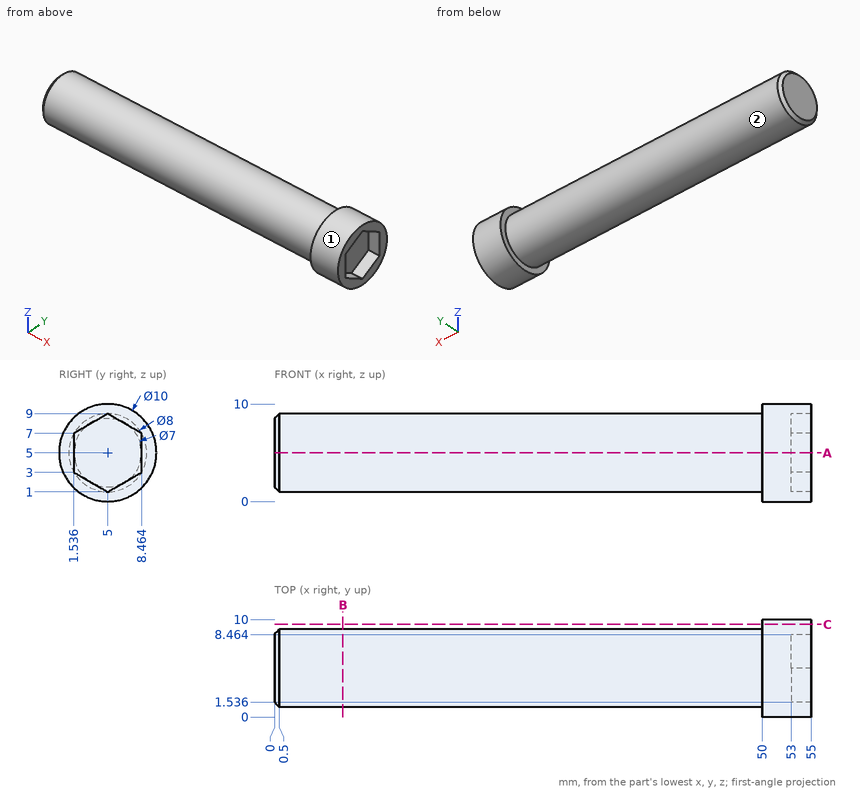
Geometry check sheet. Reference: drawing and pictorial views, mm from the part's lowest x, y, z. A direction names the side the tool comes from. Coordinates: 2 decimals unless noted, no trailing zeros. Order: outer loops, then holes, each group sorted by start corner. A loop starts at its lowest first (then second) coordinate and runs counter-clockwise, first axis right, second up. Notation, with made-up numbers: (-25, 85.25) -> (27, 85.25) arc R21 cw to (27, 110.25) -> close; hole circle Ø9 at (36, 55.25). An arc over 180 degrees is marked (long way). Use CSV: the item, a comma, the result in double quotes. Start each with the question number.
Q1. Section check B-B, the plane x = 7. Record the cut outline in (y, z).
Q2. Section check A-A, the plane z = 5. Record the cut outline in (x, y).
Q3. Tool access check on the marked faces 1 and 2. Record the directions out of +Z, -Z, +X, -X, +Y, -Y that give a thin tool (end or side, any length) a straight path to the whole face; none if there is none.
Q4. Section check C-C, the plane y = 9.5. Record the cut outline in (x, z), and give its area (3 significant figures).
Q5. Thickness scan on line 1 along X through (y, z) = (3.5, 2.25); line 2 along X through (y, z) = (9, 6.25); line 3 along Z through (x, y) = (40, 5.25). Record the ranges inside material, lowest first.
Q6. Depth check by flat-ended pin: P1, Ø2, axis at x = 16.5, y = 2.5, coming from the -Z side; P2, Ø5.5, axis at y = 4.5, z = 4, coming from the +X side; P3, Ø6, axis at x = 45, z = 5, coming from the +Y side; P4, Ø0.6, axis at x = 54.5, z = 5.5, coming from the -Y side. Enter the tip coordinate at first touch or a pass-through.
Returned:
1,outline,"circle Ø8 at (5, 5)"
2,outline,"(0, 1.5) -> (0.5, 1) -> (50, 1) -> (50, 0) -> (55, 0) -> (55, 1.54) -> (53, 1.54) -> (53, 8.46) -> (55, 8.46) -> (55, 10) -> (50, 10) -> (50, 9) -> (0.5, 9) -> (0, 8.5) -> close"
3,face 1,"+X, -X"
3,face 2,"-X"
4,outline,"(50, 2.82) -> (55, 2.82) -> (55, 7.18) -> (50, 7.18) -> close"
4,area,"21.8 mm^2"
5,line 1,"x = 0 to 53"
5,line 2,"x = 50 to 55"
5,line 3,"z = 1.01 to 8.99"
6,P1,"stops at z = 1.29"
6,P2,"stops at x = 55"
6,P3,"stops at y = 9"
6,P4,"stops at y = 0"
